```python
from build123d import *

# Parameters (mm, degrees)
F0_R     = 12.5
F1_DEPTH = 218
F2_SIZE  = 2
F4_R     = 4
F5_DEPTH = 25.001
F8_DEPTH = 135


with BuildPart() as f1:
    # F0 (on Top) → F1 (new body)
    with BuildSketch(Plane.XY):
        Circle(F0_R)
    extrude(amount=F1_DEPTH)

    # F2
    f2_edges = [f1.edges().sort_by_distance(p)[0] for p in [
        (-12.5, 0, 0),
        (-12.5, 0, 218),
    ]]
    chamfer(f2_edges, length=F2_SIZE)

    # F4 (on offset) → F5 (cut, through all)
    with BuildSketch(Plane.XZ.offset(-12.5)):
        with Locations((0, 208)):
            Circle(F4_R)
    extrude(amount=F5_DEPTH, mode=Mode.SUBTRACT)

    # F7 (on offset) → F8 (cut)
    with BuildSketch(Plane.XY.offset(52)):
        with BuildLine():
            Line((13, -1.5), (13, 1.5))
            ThreePointArc((13, 1.5), (11.5, 0), (13, -1.5))
        make_face()
    extrude(amount=F8_DEPTH, mode=Mode.SUBTRACT)


with BuildPart() as f11:
    # F10 (on offset) → F11 (revolve)
    with BuildSketch(Plane.XY.offset(48)):
        with BuildLine():
            Line((13, -1.5), (13, 1.5))
            ThreePointArc((13, 1.5), (11.5, 0), (13, -1.5))
        make_face()
    revolve(axis=Axis((13, 0, 48), (0, -1, 0)))


with BuildPart() as f1_1:
    add(f1.part)

    # F12: cut F11
    add(f11.part, mode=Mode.SUBTRACT)

    # F7 (on offset) → F13 (revolve, cut)
    with BuildSketch(Plane.XY.offset(52)):
        with BuildLine():
            Line((13, -1.5), (13, 1.5))
            ThreePointArc((13, 1.5), (11.5, 0), (13, -1.5))
        make_face()
    revolve(axis=Axis((13, 0, 52), (0, -1, 0)), mode=Mode.SUBTRACT)

    # F14 (on face) → F15 (revolve, cut)
    with BuildSketch(Plane(origin=(0, 0, 187), x_dir=(1, 0, 0), z_dir=(0, 0, -1))):
        with BuildLine():
            ThreePointArc((12.423077, 1.384615), (11.5, 0), (12.423077, -1.384615))
            Line((12.423077, -1.384615), (12.423077, 1.384615))
        make_face()
    revolve(axis=Axis((12.423077, 0, 187), (0, 1, 0)), mode=Mode.SUBTRACT)


solid = f1_1.part
```
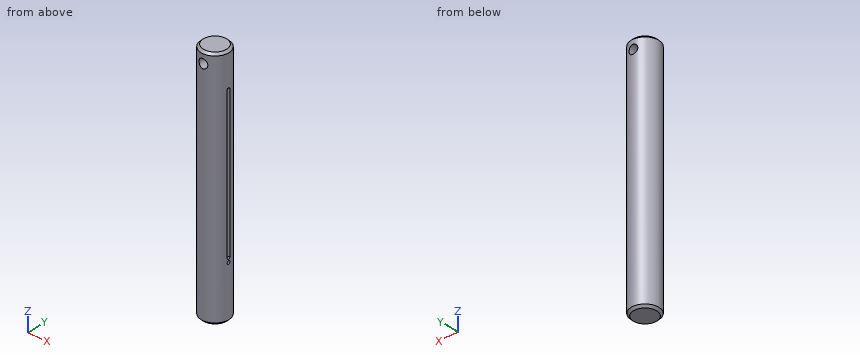
Geometry check sheet. Reference: the model listing, model coordinates, mm. Round coordinates to 2 decimals unless told otherwise and drop trailing zeros. Loops run counter-clockwise (first coordinate to the right, second up) from the corner with the lowest first, then second, coordinate; pieces in that order, holes last. Notation, with made-up numbers: (27.25, 52.5) - (82.25, 52.5) arc R14 cw to (82.25, 79.5) - close; hole circle Ø5 at (44.25, 22.25). An arc over 180 degrees is marked (long way). Write item = value, one per line. Start each with the question number.
1. Depth check by flat-ended pin: pin 1 (5 mm diameter, centred on y = 3.5, z = 127.5, fed in from +X); pin 2 (6.5 mm diameter, centred on x = 0, z = 208, fed in from +Y); pin 3 (5 mm diameter, centred on x = 8, z = 103.5, fed in from -Y) (3 decimals); pin 4 (5 mm diameter, centred on x = -6.5, z = 65, fed in from +Y). Enter the tip coordinate at first touch or a pass-through.
2. Thickness scan on line 1 (Z direction, x = 0, y = -6.5); line 2 (Y direction, x = 0.25, z = 64); line 3 (X direction, y = -1.5, z = 208). Record the ranges inside material, lowest first.
3. Section check C-C on z = 208. Enter the section's corners in (x, y), then the cut area to 3 significant figures.
4. Section check B-B on z = 151.5. Enter the section's corners in (x, y).
5. Section check A-A on x = 0. Enter the section's corners in (y, z), then the cut area to 3 significant figures.
Working result:
q1.pin_1 = 12.42
q1.pin_2 = through
q1.pin_3 = -11.225
q1.pin_4 = 11.84
q2.line_1 = 0 to 204, 212 to 218
q2.line_2 = -12.5 to 12.5
q2.line_3 = -12.41 to -4, 4 to 12.41
q3.outline = (-4, -11.84) - (-4, 11.84) arc R12.5 ccw to start; (4, -11.84) arc R12.5 ccw to (4, 11.84) - close
q3.area = 294 mm^2
q4.outline = (12.42, -1.38) arc R1.5 cw to (12.42, 1.38) arc R12.5 ccw (long way) to start
q5.outline = (-12.5, 2) - (-10.5, 0) - (10.5, 0) - (12.5, 2) - (12.5, 204) - (-12.5, 204) - close; (-12.5, 212) - (12.5, 212) - (12.5, 216) - (10.5, 218) - (-10.5, 218) - (-12.5, 216) - close
q5.area = 5,240 mm^2
